from build123d import *

# Parameters (mm, degrees)
F0_W     = 584.2
F0_H     = 219.71
F1_DEPTH = 5.334
F2_W     = 571.5
F2_H     = 213.36
F2_W_2   = 546.1
F2_H_2   = 187.96
F3_DEPTH = 12.7
F4_R     = 25.4
F6_DEPTH = 12.7
F8_DEPTH = 5.334


# Not quite as in the source:
# - a feature names something its author has since deleted; it is built from what else it names


with BuildPart() as f1:
    # F0 (on Front) → F1 (new body)
    with BuildSketch(Plane.XZ):
        with Locations((-292.1, 109.855)):
            Rectangle(F0_W, F0_H)
    extrude(amount=F1_DEPTH)

    # F2 (on face) → F3 (join)
    with BuildSketch(Plane.XZ.offset(5.334)):
        with Locations((-292.1, 113.03)):
            Rectangle(F2_W, F2_H)
        with Locations((-292.1, 113.03)):
            Rectangle(F2_W_2, F2_H_2, mode=Mode.SUBTRACT)
    extrude(amount=F3_DEPTH)

    # F4
    f4_edges = [f1.edges().sort_by_distance(p)[0] for p in [
        (-565.15, -11.684, 207.01),
        (-19.05, -11.684, 207.01),
        (-19.05, -11.684, 19.05),
        (-565.15, -11.684, 19.05),
    ]]
    fillet(f4_edges, radius=F4_R)

    # F5 (on face) → F6 (cut)
    with BuildSketch(Plane.XZ.offset(18.034)):
        Polygon((-118.11, 219.71), (-125.73, 207.01), (-118.11, 207.01), (-113.5820166854, 214.5566388576), (-110.49, 219.71), align=None)
        Polygon((-56.5979833146, 214.5566388576), (-52.07, 207.01), (-44.45, 207.01), (-52.07, 219.71), (-59.69, 219.71), align=None)
        Polygon((-59.69, 219.71), (-110.49, 219.71), (-113.5820166854, 214.5566388576), (-56.5979833146, 214.5566388576), align=None)
    extrude(amount=-F6_DEPTH, mode=Mode.SUBTRACT)

    # F7 (on face) → F8 (join)
    with BuildSketch(Plane(origin=(0, 0, 0), x_dir=(-1, 0, 0), z_dir=(0, 1, 0))):
        with BuildLine():
            Line((292.1, 0), (0, 0))
            add(Edge.make_bspline(
                [(13.97, -18.4182160117), (5.1776683434, -12.9300591082), (2.1993531585, -8.4306227348), (0, 0)],
                knots=[0.6884256157, 0.6884256157, 0.6884256157, 0.6884256157, 0.8055577438, 0.8055577438, 0.8055577438, 0.8055577438], degree=3))
            Line((13.97, -18.4182160117), (273.05, -18.4182160117))
            add(Edge.make_bspline(
                [(292.1, 0), (287.8348745006, -6.4171904537), (283.3704909948, -12.0241872437), (273.05, -18.4182160117)],
                knots=[0, 0, 0, 0, 0.1254053332, 0.1254053332, 0.1254053332, 0.1254053332], degree=3))
        make_face()
        with BuildLine():
            add(Edge.make_bspline(
                [(0, 0), (-3.4777348873, 13.330951736), (-5.0077822241, 36.49129499), (-5.08, 59.9872617497)],
                knots=[0.8055577438, 0.8055577438, 0.8055577438, 0.8055577438, 0.9907733318, 0.9907733318, 0.9907733318, 0.9907733318], degree=3))
            Line((0, 0), (0, 109.855))
            Line((0, 109.855), (-5.08, 109.855))
            Line((-5.08, 109.855), (-5.08, 63.5))
            Line((-5.08, 63.5), (-5.08, 59.9872617497))
        make_face()
        with BuildLine():
            Line((273.05, -18.4182160117), (13.97, -18.4182160117))
            add(Edge.make_bspline(
                [(143.51, -50.8), (89.8146392781, -50.5091658601), (35.101098408, -31.6082079428), (13.97, -18.4182160117)],
                knots=[0.4069154744, 0.4069154744, 0.4069154744, 0.4069154744, 0.6884256157, 0.6884256157, 0.6884256157, 0.6884256157], degree=3))
            Line((143.51, -50.8), (146.0426574413, -50.8))
            add(Edge.make_bspline(
                [(273.05, -18.4182160117), (250.2469136161, -32.545798741), (198.8550496381, -50.5155722463), (146.0426574413, -50.8)],
                knots=[0.1254053332, 0.1254053332, 0.1254053332, 0.1254053332, 0.4024879494, 0.4024879494, 0.4024879494, 0.4024879494], degree=3))
        make_face()
        with BuildLine():
            Line((584.2, 0), (292.1, 0))
            add(Edge.make_bspline(
                [(292.1, 0), (295.2511238563, -6.7739107165), (300.4280406329, -12.1526213408), (311.15, -18.4182160117)],
                knots=[0, 0, 0, 0, 0.1254053332, 0.1254053332, 0.1254053332, 0.1254053332], degree=3))
            Line((311.15, -18.4182160117), (570.23, -18.4182160117))
            add(Edge.make_bspline(
                [(570.23, -18.4182160117), (579.0383616328, -12.9277742975), (582.0053728244, -8.4368679309), (584.2, 0)],
                knots=[0.6884256157, 0.6884256157, 0.6884256157, 0.6884256157, 0.8055577438, 0.8055577438, 0.8055577438, 0.8055577438], degree=3))
        make_face()
        with BuildLine():
            Line((-5.08, 109.855), (0, 109.855))
            Line((0, 109.855), (0, 219.71))
            add(Edge.make_bspline(
                [(0, 219.71), (-3.3633398359, 214.4958413315), (-4.221669918, 209.4829206658), (-5.08, 204.47)],
                knots=[0.8528806378, 0.8528806378, 0.8528806378, 0.8528806378, 1, 1, 1, 1], degree=3))
            Line((-5.08, 204.47), (-5.08, 109.855))
        make_face()
        with BuildLine():
            Line((570.23, -18.4182160117), (311.15, -18.4182160117))
            add(Edge.make_bspline(
                [(311.15, -18.4182160117), (334.9383025593, -32.3193936455), (386.0216290424, -50.5861863086), (438.8223695347, -50.8)],
                knots=[0.1254053332, 0.1254053332, 0.1254053332, 0.1254053332, 0.4036361962, 0.4036361962, 0.4036361962, 0.4036361962], degree=3))
            Line((438.8223695347, -50.8), (440.69, -50.8))
            add(Edge.make_bspline(
                [(440.69, -50.8), (494.1504250391, -50.5826159423), (549.0603758608, -31.6136991551), (570.23, -18.4182160117)],
                knots=[0.4069154744, 0.4069154744, 0.4069154744, 0.4069154744, 0.6884256157, 0.6884256157, 0.6884256157, 0.6884256157], degree=3))
        make_face()
        with BuildLine():
            Line((584.2, 109.855), (584.2, 0))
            add(Edge.make_bspline(
                [(584.2, 0), (587.6660611317, 13.3246778013), (589.2055548561, 36.4918183962), (589.28, 59.9101174948)],
                knots=[0.8055577438, 0.8055577438, 0.8055577438, 0.8055577438, 0.9905491269, 0.9905491269, 0.9905491269, 0.9905491269], degree=3))
            Line((589.28, 59.9101174948), (589.28, 63.5))
            Line((589.28, 63.5), (589.28, 109.855))
            Line((589.28, 109.855), (584.2, 109.855))
        make_face()
        with BuildLine():
            add(Edge.make_bspline(
                [(8.9497229668, 229.3903513516), (5.0117556013, 226.1203537614), (2.0435071593, 222.8780326962), (0, 219.71)],
                knots=[0.7634934559, 0.7634934559, 0.7634934559, 0.7634934559, 0.8528806378, 0.8528806378, 0.8528806378, 0.8528806378], degree=3))
            Line((0, 219.71), (292.1, 219.71))
            Line((292.1, 219.71), (8.9497229668, 229.3903513516))
        make_face()
        with BuildLine():
            Line((584.2, 219.71), (584.2, 109.855))
            Line((584.2, 109.855), (589.28, 109.855))
            Line((589.28, 109.855), (589.28, 204.47))
            add(Edge.make_bspline(
                [(584.2, 219.71), (587.5633398359, 214.4958413315), (588.421669918, 209.4829206658), (589.28, 204.47)],
                knots=[0.8528806378, 0.8528806378, 0.8528806378, 0.8528806378, 1, 1, 1, 1], degree=3))
        make_face()
        with BuildLine():
            add(Edge.make_bspline(
                [(9.5340725562, 229.87), (9.3369695017, 229.7100546344), (9.1421880555, 229.5501699377), (8.9497229668, 229.3903513516)],
                knots=[0.759124727, 0.759124727, 0.759124727, 0.759124727, 0.7634934559, 0.7634934559, 0.7634934559, 0.7634934559], degree=3))
            Line((8.9497229668, 229.3903513516), (292.1, 219.71))
            Line((292.1, 219.71), (575.2502770332, 229.3903513516))
            add(Edge.make_bspline(
                [(574.6659274438, 229.87), (574.8630304983, 229.7100546344), (575.0578119445, 229.5501699377), (575.2502770332, 229.3903513516)],
                knots=[0.759124727, 0.759124727, 0.759124727, 0.759124727, 0.7634934559, 0.7634934559, 0.7634934559, 0.7634934559], degree=3))
            Line((574.6659274438, 229.87), (539.75, 229.87))
            Line((539.75, 229.87), (292.1, 229.87))
            Line((292.1, 229.87), (44.45, 229.87))
            Line((44.45, 229.87), (9.5340725562, 229.87))
        make_face()
        with BuildLine():
            Line((575.2502770332, 229.3903513516), (292.1, 219.71))
            Line((292.1, 219.71), (584.2, 219.71))
            add(Edge.make_bspline(
                [(575.2502770332, 229.3903513516), (579.1882443987, 226.1203537614), (582.1564928407, 222.8780326962), (584.2, 219.71)],
                knots=[0.7634934559, 0.7634934559, 0.7634934559, 0.7634934559, 0.8528806378, 0.8528806378, 0.8528806378, 0.8528806378], degree=3))
        make_face()
        with BuildLine():
            add(Edge.make_bspline(
                [(44.45, 248.92), (28.9100061464, 242.7028057711), (17.3818410687, 236.2383143168), (9.5340725562, 229.87)],
                knots=[0.5851813382, 0.5851813382, 0.5851813382, 0.5851813382, 0.759124727, 0.759124727, 0.759124727, 0.759124727], degree=3))
            Line((9.5340725562, 229.87), (44.45, 229.87))
            Line((44.45, 229.87), (44.45, 248.92))
        make_face()
        with BuildLine():
            Line((44.45, 248.92), (44.45, 229.87))
            Line((44.45, 229.87), (292.1, 229.87))
            Line((292.1, 229.87), (292.1, 306.07))
            add(Edge.make_bspline(
                [(292.1, 306.07), (194.4148678752, 287.9529601014), (96.7297357504, 269.8359202028), (44.45, 248.92)],
                knots=[0, 0, 0, 0, 0.5851813382, 0.5851813382, 0.5851813382, 0.5851813382], degree=3))
        make_face()
        with BuildLine():
            Line((539.75, 229.87), (574.6659274438, 229.87))
            add(Edge.make_bspline(
                [(539.75, 248.92), (555.2899938536, 242.7028057711), (566.8181589313, 236.2383143168), (574.6659274438, 229.87)],
                knots=[0.5851813382, 0.5851813382, 0.5851813382, 0.5851813382, 0.759124727, 0.759124727, 0.759124727, 0.759124727], degree=3))
            Line((539.75, 248.92), (539.75, 229.87))
        make_face()
        with BuildLine():
            Line((292.1, 306.07), (292.1, 229.87))
            Line((292.1, 229.87), (539.75, 229.87))
            Line((539.75, 229.87), (539.75, 248.92))
            add(Edge.make_bspline(
                [(292.1, 306.07), (389.7851321248, 287.9529601014), (487.4702642496, 269.8359202028), (539.75, 248.92)],
                knots=[0, 0, 0, 0, 0.5851813382, 0.5851813382, 0.5851813382, 0.5851813382], degree=3))
        make_face()
    extrude(amount=-F8_DEPTH)


solid = f1.part
Check sheet for the modelled part. Datum: model origin and axes. Units: mm. A direction names the side the tool comes from. Round coordinates to 2 decimals unless told otherwise and drop trailing zeros. Loops run counter-clockwise (first coordinate to the right, second up) from the corner with the lowest first, then second, coordinate; pieces in that order, holes last. Notation, with made-up numbers: (23, 31.5) -> (49, 31.5) arc R16 cw to (49, 55.5) -> close; hole circle Ø6 at (2.5, -36.75). An arc over 180 degrees is marked (long way). Put each result on its own line as item: value. Start each with the question number.
1. Section check B-B (z = 171). Enter the section's corners in (x, y), plus the area to 3 significant figures.
2. Draft check along X on faces 1 (the face through (-6.35, -12, 112)), 2 (the face through (-314.6, -18.034, 18.7)), 3 (the face through (-86, -12, 207.01)). Enter one of: +X half, -X half, draft (parallel to the pull), parting line (faces both ways), or undercut.
3. Gauge pin test, flat ends, axial feed: pin 1 (4 mm diameter, centred on x = -281.5, y = -12, fed in from -Z); pin 2 (6 mm diameter, centred on x = -431, z = 154.5, fed in from -Y); pin 3 (6.5 mm diameter, centred on x = -32.5, y = -13.5, fed in from +Z). Record the tip position at first contact, or that the pin passes through.
4. Scan lines: probe 1 along Z at (x, y) = (-430, -13); probe 2 along X at (y, z) = (-12.75, 49); probe 3 along Y at (x, z) = (-378.5, 60). Record each from-to range of solid material in increasing order.
5. Section check A-A (y = -8.75). Enter the section's corners in (x, z).
6. Access from +Z, -Z, +X, -X, +Y, -Y to the whole of each face (thin tool, end or side, straight path). Record for faces 4 (the face through (-351, -12, 219.71)), 5 (the face through (-296, -12, 6.35)), 6 (the face through (-26.69, -11.77, 26.29)).
Findings:
1. outline: (-589.28, -5.33) -> (-577.85, -5.33) -> (-577.85, -18.03) -> (-565.15, -18.03) -> (-565.15, -5.33) -> (-19.05, -5.33) -> (-19.05, -18.03) -> (-6.35, -18.03) -> (-6.35, -5.33) -> (5.08, -5.33) -> (5.08, 0) -> (-589.28, 0) -> close
1. area: 3,490 mm^2
2. face 1: +X half
2. face 2: draft
2. face 3: undercut
3. pin 1: stops at z = 6.35
3. pin 2: stops at y = -5.33
3. pin 3: stops at z = 219.71
4. probe 1: z = 6.35 to 19.05, 207.01 to 219.71
4. probe 2: x = -577.85 to -565.15, -19.05 to -6.35
4. probe 3: y = -5.33 to 0
5. outline: (-577.85, 6.35) -> (-6.35, 6.35) -> (-6.35, 219.71) -> (-52.07, 219.71) -> (-44.45, 207.01) arc R25.4 cw to (-19.05, 181.61) -> (-19.05, 44.45) arc R25.4 cw to (-44.45, 19.05) -> (-539.75, 19.05) arc R25.4 cw to (-565.15, 44.45) -> (-565.15, 181.61) arc R25.4 cw to (-539.75, 207.01) -> (-125.73, 207.01) -> (-118.11, 219.71) -> (-577.85, 219.71) -> close; (-118.11, 207.01) -> (-52.07, 207.01) -> (-56.6, 214.56) -> (-113.58, 214.56) -> close
6. face 4: +Z, +X, -X, -Y
6. face 5: -Z, +X, -X, -Y
6. face 6: -Y
